Design review of the part built by this model. Coordinates are the model's own, in mm. Face numbers are marked on the shaded views. A direction names the side the tool comes from. Coordinates: 2 decimals unless noted, no trailing zeros. Loops run counter-clockwise (first coordinate to the right, second up) from the corner with the lowest first, then second, coordinate; pieces in that order, holes last.
Q1. Draft analysis for pull direction Z (two halves, no side actions). For the marked faces 1, 2 and 3, state which applies: released by +Z, released by -Z, zero draft, split by the parting line, or undercut.
Q2. For P1, Ø4, axis at x = -5.5, y = 17, coming from the -Z side; P2, Ø5, axis at x = -16.5, y = 15.5, coming from the +Z side; P3, Ø10, axis at x = 10.5, y = -7, coming from the +Z side; P4, Ø1, axis at x = -9, z = 28, coming from the +Y side, all flat-tipped, find the tip position at first contact; note any pin that passes through.
Q3. Machinability: for the marked faces 4, 5 and 6, which of the approach directions +Z, -Z, +X, -X, +Y, -Y give a long, thin tool a straight path to every point of the face, cutting with its end or side? Answer none if there is none.
Q4. Add section C-C on x = 10. Give the boundary of the cut face in (y, z), and give its area (3 significant figures).
Q5. Add section A-A on y = 34. Give the boundary of the cut face in (x, z).
Q6. Wall thickness on probe 1 along X at (y, z) = (15, 1.4); probe 2 along Y at (x, z) = (17.5, 1.9); probe 3 along X at (y, z) = (34, 48.55): over which ranges is each line inside the solid? List them lowest first.
Q7. Add section D-D on x = -1.5. Give the boundary of the cut face in (y, z), and give its area (3 significant figures).
Q8. Add section B-B on x = 17.5. Give the number of separate pieces and of enclosed holes in the cut face, and give its area (3 significant figures).
```python
from build123d import *

# Parameters (mm, degrees)
SKETCH1_W           = 55
SKETCH1_H           = 50
SKETCH1_R           = 2.5
BOSS_EXTRUDE1_DEPTH = 5
SKETCH2_R           = 5
CUT_EXTRUDE1_DEPTH  = 2
SKETCH3_W           = 55
SKETCH3_H           = 52
BOSS_EXTRUDE2_DEPTH = 16
SKETCH4_R           = 4.1
CUT_EXTRUDE2_DEPTH  = 17
BOSS_EXTRUDE3_DEPTH = 5
SKETCH6_W           = 45
SKETCH6_H           = 40
CUT_EXTRUDE3_DEPTH  = 12
SKETCH8_R           = 2.5
CUT_EXTRUDE5_DEPTH  = 5
SKETCH10_R          = 5
CUT_EXTRUDE6_DEPTH  = 2


with BuildPart() as part:
    # Sketch1 → Boss-Extrude1 (new body)
    with BuildSketch(Plane.XY):
        Rectangle(SKETCH1_W, SKETCH1_H)
        with Locations((-17.5, -15)):
            Circle(SKETCH1_R, mode=Mode.SUBTRACT)
        with Locations((17.5, -15)):
            Circle(SKETCH1_R, mode=Mode.SUBTRACT)
        with Locations((17.5, 15)):
            Circle(SKETCH1_R, mode=Mode.SUBTRACT)
        with Locations((-17.5, 15)):
            Circle(SKETCH1_R, mode=Mode.SUBTRACT)
    extrude(amount=BOSS_EXTRUDE1_DEPTH)

    # Sketch2 → Cut-Extrude1 (cut)
    with BuildSketch(Plane.XY.offset(5)):
        with Locations((-17.5, -15)):
            Circle(SKETCH2_R)
        with Locations((17.5, -15)):
            Circle(SKETCH2_R)
        with Locations((-17.5, 15)):
            Circle(SKETCH2_R)
        with Locations((17.5, 15)):
            Circle(SKETCH2_R)
    extrude(amount=-CUT_EXTRUDE1_DEPTH, mode=Mode.SUBTRACT)

    # Sketch3 → Boss-Extrude2 (add)
    with BuildSketch(Plane(origin=(0, 25, 0), x_dir=(1, 0, 0), z_dir=(0, 1, 0))):
        with Locations((0, -26)):
            Rectangle(SKETCH3_W, SKETCH3_H)
    extrude(amount=BOSS_EXTRUDE2_DEPTH)

    # Sketch4 → Cut-Extrude2 (cut, through all)
    with BuildSketch(Plane(origin=(0, 25, 0), x_dir=(-1, 0, 0), z_dir=(0, -1, 0))):
        with Locations((0, -27)):
            Circle(SKETCH4_R)
    extrude(amount=-CUT_EXTRUDE2_DEPTH, mode=Mode.SUBTRACT)

    # Sketch5 → Boss-Extrude3 (add)
    with BuildSketch(Plane.ZY.offset(27.5)):
        with BuildLine():
            Line((5, -25), (5, 25))
            Line((5, 25), (52, 25))
            add(Edge.make_bspline(
                [(52, 25), (52, 4.232970162), (15.26663468, -20.719918254), (5, -25)],
                knots=[0, 0, 0, 0, 0.911487557, 0.911487557, 0.911487557, 0.911487557], degree=3))
        make_face()
    boss_extrude3 = extrude(amount=-BOSS_EXTRUDE3_DEPTH)

    # Mirror1: Boss-Extrude3 across plane
    add(boss_extrude3.mirror(Plane(origin=(0, 0, 0), x_dir=(0, 0, 1), z_dir=(1, 0, 0))))

    # Sketch6 → Cut-Extrude3 (cut)
    with BuildSketch(Plane(origin=(0, 41, 0), x_dir=(1, 0, 0), z_dir=(0, 1, 0))):
        with Locations((0, -27)):
            Rectangle(SKETCH6_W, SKETCH6_H)
    extrude(amount=-CUT_EXTRUDE3_DEPTH, mode=Mode.SUBTRACT)

    # Sketch8 → Cut-Extrude5 (cut)
    with BuildSketch(Plane.XY.offset(52)):
        with Locations((16, 34)):
            Circle(SKETCH8_R)
        with Locations((-16, 34)):
            Circle(SKETCH8_R)
    extrude(amount=-CUT_EXTRUDE5_DEPTH, mode=Mode.SUBTRACT)

    # Sketch10 → Cut-Extrude6 (cut)
    with BuildSketch(Plane(origin=(0, 0, 47), x_dir=(-1, 0, 0), z_dir=(0, 0, -1))):
        with Locations((-16, 34)):
            Circle(SKETCH10_R)
        with Locations((16, 34)):
            Circle(SKETCH10_R)
    extrude(amount=-CUT_EXTRUDE6_DEPTH, mode=Mode.SUBTRACT)


solid = part.part
```
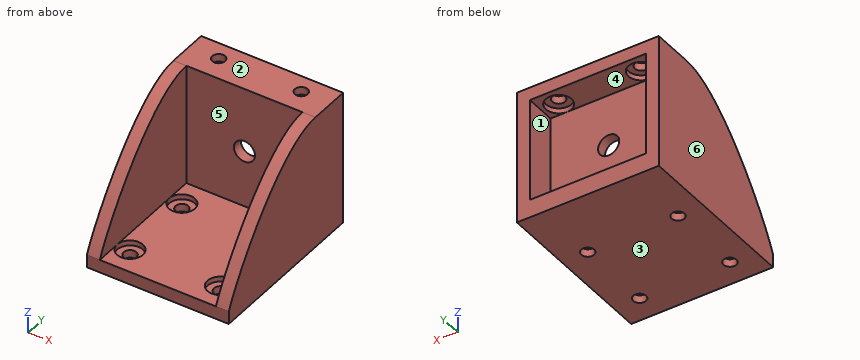
Entries:
1. face 1: undercut
1. face 2: released by +Z
1. face 3: released by -Z
2. P1: stops at z = 0
2. P2: stops at z = 3
2. P3: stops at z = 5
2. P4: stops at y = 29
3. face 4: +Y
3. face 5: +Z, -Y
3. face 6: +Z, -Z, -X, +Y, -Y
4. outline: (-25, 0) - (41, 0) - (41, 7) - (29, 7) - (29, 47) - (41, 47) - (41, 52) - (25, 52) - (25, 5) - (-25, 5) - close
4. area: 602 mm2
5. outline: (-27.5, 0) - (27.5, 0) - (27.5, 52) - (18.5, 52) - (18.5, 49) - (21, 49) - (21, 47) - (22.5, 47) - (22.5, 7) - (-22.5, 7) - (-22.5, 47) - (-21, 47) - (-21, 49) - (-18.5, 49) - (-18.5, 52) - (-27.5, 52) - close; (-13.5, 49) - (-11, 49) - (-11, 47) - (11, 47) - (11, 49) - (13.5, 49) - (13.5, 52) - (-13.5, 52) - close
6. probe 1: x = -27.5 to -20, -15 to 15, 20 to 27.5
6. probe 2: y = -25 to -17.5, -12.5 to 12.5, 17.5 to 41
6. probe 3: x = -27.5 to -21, -11 to 11, 21 to 27.5
7. outline: (-25, 0) - (41, 0) - (41, 7) - (29, 7) - (29, 23.18) - (25, 23.18) - (25, 5) - (-25, 5) - close; (25, 30.82) - (29, 30.82) - (29, 47) - (41, 47) - (41, 52) - (25, 52) - close
7. area: 571 mm2
8. separate pieces: 4
8. enclosed holes: 0
8. area: 501 mm2
